The drawing under review shows one solid part. Ordinate dimensions are in mm from its lowest x, y, z. Round coordinates to 2 decimals unless told otherwise and drop trailing zeros. Order: outer loops, then holes, each group sorted by start corner. A loop starts at its lowest first (then second) coordinate and runs counter-clockwise, first axis right, second up. Notation, with made-up numbers: (61.25, -27) - (85.25, -27) arc R7 ccw to (85.25, -16) - close; hole circle Ø10 at (-33.75, 64.25). An arc over 180 degrees is marked (long way). One line per question, with ' | ' between items.
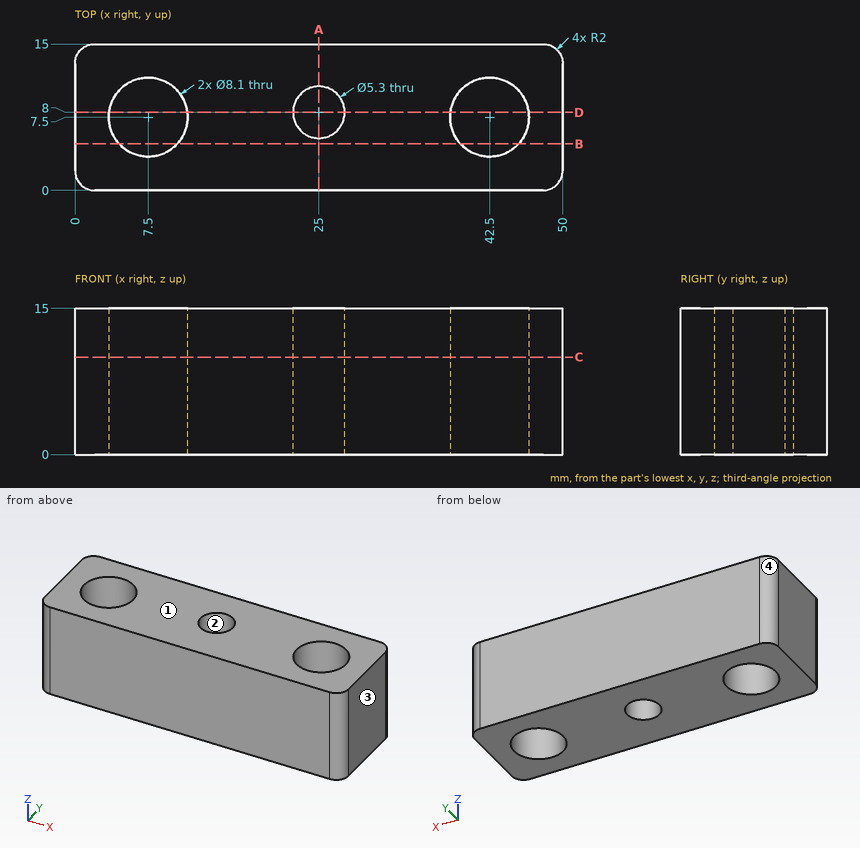
(1) We need section A-A on x = 25. State the section outline as (y, z) points.
Output values:
outline: (0, 0) - (5.35, 0) - (5.35, 15) - (0, 15) - close; (10.65, 0) - (15, 0) - (15, 15) - (10.65, 15) - close
(2) We need section C-C on z = 10. State the section outline as (x, y) points.
Output values:
outline: (0, 2) arc R2 ccw to (2, 0) - (48, 0) arc R2 ccw to (50, 2) - (50, 13) arc R2 ccw to (48, 15) - (2, 15) arc R2 ccw to (0, 13) - close; hole circle Ø8.1 at (7.5, 7.5); hole circle Ø5.3 at (25, 8); hole circle Ø8.1 at (42.5, 7.5)
(3) We need section D-D on y = 8. State the section outline as (x, z) points.
Output values:
outline: (0, 0) - (3.48, 0) - (3.48, 15) - (0, 15) - close; (11.52, 0) - (22.35, 0) - (22.35, 15) - (11.52, 15) - close; (27.65, 0) - (38.48, 0) - (38.48, 15) - (27.65, 15) - close; (46.52, 0) - (50, 0) - (50, 15) - (46.52, 15) - close
(4) We need section B-B on y = 4.75. State the section outline as (x, z) points.
Output values:
outline: (0, 0) - (4.53, 0) - (4.53, 15) - (0, 15) - close; (10.47, 0) - (39.53, 0) - (39.53, 15) - (10.47, 15) - close; (45.47, 0) - (50, 0) - (50, 15) - (45.47, 15) - close
(5) For probe 1 along Y at (x, z) = (25, 8); probe 2 along X at (y, z) = (7.5, 10.5); probe 3 along Y at (x, z) = (7.5, 12.25), list the stretches that pass through material, from the lowest coordinate up. Write a range as [from, to].
Output values:
probe 1: [0, 5.35], [10.65, 15] | probe 2: [0, 3.45], [11.55, 22.4], [27.6, 38.45], [46.55, 50] | probe 3: [0, 3.45], [11.55, 15]
(6) Mouldability with a two-part tool opening along X and no side actions: class the marked faces 1, 2, 3 and 4 as released by +X, released by -X, zero draft, split by the parting line, or undercut.
Output values:
face 1: zero draft | face 2: undercut | face 3: released by +X | face 4: released by -X
